from build123d import *

# Parameters (mm, degrees)
SALIENTE_EXTRUIR1_DEPTH = 50.8
CROQUIS2_R              = 3.175
CORTAR_EXTRUIR1_DEPTH   = 96.038097624


with BuildPart() as part:
    # Croquis1 → Saliente-Extruir1 (new, symmetric)
    with BuildSketch(Plane(origin=(0, 0, 0), x_dir=(0, 0, -1), z_dir=(1, 0, 0))):
        Polygon((0, 76.2), (0, 0), (25.4, 0), (25.4, 3), (3, 3), (3, 76.2), align=None)
    extrude(amount=SALIENTE_EXTRUIR1_DEPTH, both=True)

    # Croquis2 → Cortar-Extruir1 (cut, through all)
    with BuildSketch(Plane.XY):
        with Locations((-4.334249313, 32.6)):
            Circle(CROQUIS2_R)
        with BuildLine():
            Line((42.015750687, 26.25), (12.015750687, 26.25))
            ThreePointArc((12.015750687, 26.25), (5.665750687, 32.6), (12.015750687, 38.95))
            Line((12.015750687, 38.95), (42.015750687, 38.95))
            ThreePointArc((42.015750687, 38.95), (48.365750687, 32.6), (42.015750687, 26.25))
        make_face()
    extrude(amount=-CORTAR_EXTRUIR1_DEPTH, mode=Mode.SUBTRACT)


solid = part.part
The listing builds one solid part. Answer for the finished solid, in the listing's coordinates (mm). A direction names the side the tool comes from. Coordinates: 2 decimals unless noted, no trailing zeros. Loops run counter-clockwise (first coordinate to the right, second up) from the corner with the lowest first, then second, coordinate; pieces in that order, holes last.
1) Find section C-C on z = -17.25. Write down the section's boundary in (x, y), then the cut area to 3 significant figures.
2) A tool of negligible diameter and unlimited length cuts with its end or side. For faces 5 (the face through (27, 26.25, -1)), 6 (the face through (1, 39, -3)), 7 (the face through (1, 39, 0)), from which of +Z, -Z, +X, -X, +Y, -Y can it reach the whole face along a straight path? Write none if from no direction.
3) Find section A-A on y = 32.6. Write down the section's boundary in (x, z).
4) Determine the mould class of faces 1 (the face through (-50.8, 30, -2)), 2 (the face through (-5.02, 29.5, -1.48)), 3 (the face through (1, 1, -25.4)), 4 (the face through (5.667, 32.46, -1.479)) for opening direction X: pulls with the +X half, pulls with the -X half, needs draft (parallel to the pull), parting line crosses it, or undercut.
5) Find section B-B on x = 10.5. Write down the section's boundary in (y, z), then the cut area to 3 significant figures.
6) A flat-ended cylindrical pin translates along its axis: pin 1 Ø5 at (x, y) = (-25, 15) entering from -Z. Find the tip coordinate at first contact, or state that the pin passes through.
7) Find section D-D on y = 21.5. Write down the section's boundary in (x, z), then the cut area to 3 significant figures.
8) Find the intervals of material crossed by L1, parallel to Y at x = -33, z = -14.75; L2, parallel to Z at x = -26.5, y = 61, in increasing order.
Values:
1. outline: (-50.8, 0) - (50.8, 0) - (50.8, 3) - (-50.8, 3) - close
1. area: 305 mm2
2. face 5: +Z, -Z
2. face 6: -Z, +X, -X, +Y
2. face 7: +Z, +X, -X, +Y, -Y
3. outline: (-50.8, -3) - (-7.51, -3) - (-7.51, 0) - (-50.8, 0) - close; (-1.16, -3) - (5.67, -3) - (5.67, 0) - (-1.16, 0) - close; (48.37, -3) - (50.8, -3) - (50.8, 0) - (48.37, 0) - close
4. face 1: pulls with the -X half
4. face 2: undercut
4. face 3: needs draft
4. face 4: undercut
5. outline: (0, -25.4) - (3, -25.4) - (3, -3) - (26.43, -3) - (26.43, 0) - (0, 0) - close; (38.77, -3) - (76.2, -3) - (76.2, 0) - (38.77, 0) - close
5. area: 259 mm2
6. pin 1: stops at z = -3
7. outline: (-50.8, -3) - (50.8, -3) - (50.8, 0) - (-50.8, 0) - close
7. area: 305 mm2
8. L1: y = 0 to 3
8. L2: z = -3 to 0
